```python
from build123d import *

# Parameters (mm, degrees)
F0_R     = 279.4
F1_DEPTH = 101.6
F2_R     = 12.7
F2_R_2   = 12.5
F3_DEPTH = 50.8


with BuildPart() as f1:
    # F0 (on Top) → F1 (new body)
    with BuildSketch(Plane.XY):
        with BuildLine():
            ThreePointArc((165.1, -285.961588), (285.961588, -165.1), (330.2, 0))
            ThreePointArc((330.2, 0), (316.035905, 95.673125), (274.758772, 183.138356))
            ThreePointArc((274.758772, 183.138356), (225.85856, 240.873309), (165.1, 285.961588))
            ThreePointArc((165.1, 285.961588), (-95.673125, 316.035905), (-295.981854, 146.378898))
            ThreePointArc((-295.981854, 146.378898), (-321.531685, 75.162596), (-330.2, 0))
            ThreePointArc((-330.2, 0), (-225.85856, -240.873309), (21.223083, -329.517254))
            ThreePointArc((21.223083, -329.517254), (95.673125, -316.035905), (165.1, -285.961588))
        make_face()
        Circle(F0_R, mode=Mode.SUBTRACT)
        with BuildLine():
            ThreePointArc((165.1, 285.961588), (225.85856, 240.873309), (274.758772, 183.138356))
            ThreePointArc((274.758772, 183.138356), (419.955029, 555.806639), (346.296428, 948.919871))
            ThreePointArc((346.296428, 948.919871), (343.096456, 900.151785), (327.593656, 853.80279))
            ThreePointArc((327.593656, 853.80279), (346.365994, 854.936106), (365.172292, 855.026849))
            Line((365.172292, 855.026849), (386.159106, 781.773906))
            ThreePointArc((386.159106, 781.773906), (330.519346, 792.374089), (274.106758, 787.298))
            ThreePointArc((274.106758, 787.298), (233.337853, 773.127606), (196.453349, 750.712498))
            ThreePointArc((196.453349, 750.712498), (183.140497, 739.629863), (170.813812, 727.459832))
            Line((170.813812, 727.459832), (159.193876, 746.42974))
            ThreePointArc((159.193876, 746.42974), (148.199724, 746.572871), (137.232142, 747.350049))
            ThreePointArc((137.232142, 747.350049), (210.182068, 520.220384), (165.1, 285.961588))
        make_face()
        with BuildLine():
            ThreePointArc((219.740654, 389.881855), (289.102738, 373.429577), (335.428058, 319.247098))
            Line((335.428058, 319.247098), (315.070275, 279.674231))
            ThreePointArc((315.070275, 279.674231), (278.207397, 339.338206), (208.315586, 345.151683))
            Line((208.315586, 345.151683), (219.740654, 389.881855))
        make_face(mode=Mode.SUBTRACT)
        with BuildLine():
            ThreePointArc((230.090316, 495.358171), (318.97663, 501.347432), (378.566059, 435.122451))
            Line((378.566059, 435.122451), (364.622182, 390.380044))
            ThreePointArc((364.622182, 390.380044), (308.575729, 448.660988), (227.861751, 443.851925))
            Line((227.861751, 443.851925), (230.090316, 495.358171))
        make_face(mode=Mode.SUBTRACT)
        with BuildLine():
            ThreePointArc((220.506904, 588.747772), (315.233937, 615.350933), (401.950913, 568.863247))
            Line((401.950913, 568.863247), (395.450001, 513.362684))
            ThreePointArc((395.450001, 513.362684), (315.191991, 550.934084), (228.323604, 533.417188))
            Line((228.323604, 533.417188), (220.506904, 588.747772))
        make_face(mode=Mode.SUBTRACT)
        with BuildLine():
            ThreePointArc((190.731506, 685.758289), (287.267753, 744.917108), (397.553807, 719.304627))
            Line((397.553807, 719.304627), (403.311044, 656.066156))
            ThreePointArc((403.311044, 656.066156), (302.181037, 674.537443), (211.661495, 625.806762))
            Line((211.661495, 625.806762), (190.731506, 685.758289))
        make_face(mode=Mode.SUBTRACT)
        with BuildLine():
            ThreePointArc((578.608057, -492.521545), (345.433034, -442.133203), (165.1, -285.961588))
            ThreePointArc((165.1, -285.961588), (95.673125, -316.035905), (21.223083, -329.517254))
            ThreePointArc((21.223083, -329.517254), (271.365154, -641.595043), (648.6405, -774.36144))
            ThreePointArc((648.6405, -774.36144), (608.006084, -747.206139), (575.618078, -710.605824))
            ThreePointArc((575.618078, -710.605824), (567.21339, -727.429803), (557.888826, -743.761906))
            Line((557.888826, -743.761906), (483.95651, -725.310549))
            ThreePointArc((483.95651, -725.310549), (520.956418, -682.425195), (544.76669, -631.032416))
            ThreePointArc((544.76669, -631.032416), (552.879221, -588.640311), (551.90942, -545.489839))
            ThreePointArc((551.90942, -545.489839), (548.968002, -528.419254), (544.591788, -511.659017))
            Line((544.591788, -511.659017), (566.830179, -511.080811))
            ThreePointArc((566.830179, -511.080811), (572.45121, -501.631161), (578.608057, -492.521545))
        make_face()
        with BuildLine():
            ThreePointArc((227.777264, -385.241916), (178.848131, -437.085104), (108.762068, -450.112768))
            Line((108.762068, -450.112768), (84.669851, -412.695977))
            ThreePointArc((84.669851, -412.695977), (154.771808, -410.603776), (194.752332, -352.982431))
            Line((194.752332, -352.982431), (227.777264, -385.241916))
        make_face(mode=Mode.SUBTRACT)
        with BuildLine():
            ThreePointArc((313.947602, -446.943144), (274.691297, -526.915581), (187.544067, -545.40905))
            Line((187.544067, -545.40905), (155.767944, -510.962094))
            ThreePointArc((155.767944, -510.962094), (234.263949, -491.564914), (270.456167, -419.260027))
            Line((270.456167, -419.260027), (313.947602, -446.943144))
        make_face(mode=Mode.SUBTRACT)
        with BuildLine():
            ThreePointArc((399.617075, -485.338467), (375.292572, -580.676064), (291.674567, -632.531325))
            Line((291.674567, -632.531325), (246.860125, -599.151088))
            ThreePointArc((246.860125, -599.151088), (319.526917, -548.431313), (347.791033, -464.442635))
            Line((347.791033, -464.442635), (399.617075, -485.338467))
        make_face(mode=Mode.SUBTRACT)
        with BuildLine():
            ThreePointArc((498.518346, -508.057474), (501.483263, -621.239726), (424.159177, -703.94401))
            Line((424.159177, -703.94401), (366.514436, -677.310688))
            ThreePointArc((366.514436, -677.310688), (433.076043, -598.965176), (436.133807, -496.207613))
            Line((436.133807, -496.207613), (498.518346, -508.057474))
        make_face(mode=Mode.SUBTRACT)
        with BuildLine():
            ThreePointArc((327.593656, 853.80279), (343.096456, 900.151785), (346.296428, 948.919871))
            ThreePointArc((346.296428, 948.919871), (23.952295, 1074.045306), (137.232142, 747.350049))
            ThreePointArc((137.232142, 747.350049), (148.199724, 746.572871), (159.193876, 746.42974))
            Line((159.193876, 746.42974), (140.616896, 776.757238))
            ThreePointArc((140.616896, 776.757238), (228.227479, 829.544451), (327.593656, 853.80279))
        make_face()
        Polygon((75.530644, 936.905829), (115.853144, 1006.746447), (196.498144, 1006.746447), (236.820644, 936.905829), (196.498144, 867.06521), (115.853144, 867.06521), align=None, mode=Mode.SUBTRACT)
        with BuildLine():
            ThreePointArc((648.6405, -774.36144), (918.174372, -557.765949), (578.608057, -492.521545))
            ThreePointArc((578.608057, -492.521545), (572.45121, -501.631161), (566.830179, -511.080811))
            Line((566.830179, -511.080811), (602.383053, -510.156423))
            ThreePointArc((602.383053, -510.156423), (604.292829, -612.42302), (575.618078, -710.605824))
            ThreePointArc((575.618078, -710.605824), (608.006084, -747.206139), (648.6405, -774.36144))
        make_face()
        Polygon((773.618927, -533.864371), (813.941427, -603.704989), (773.618927, -673.545608), (692.973927, -673.545608), (652.651427, -603.704989), (692.973927, -533.864371), align=None, mode=Mode.SUBTRACT)
        with BuildLine():
            ThreePointArc((-330.2, 0), (-321.531685, 75.162596), (-295.981854, 146.378898))
            ThreePointArc((-295.981854, 146.378898), (-691.320184, 85.788404), (-994.936929, -174.558431))
            ThreePointArc((-994.936929, -174.558431), (-951.102541, -152.945645), (-903.211734, -143.196967))
            ThreePointArc((-903.211734, -143.196967), (-913.579384, -127.506303), (-923.061118, -111.264943))
            Line((-923.061118, -111.264943), (-870.115616, -56.463358))
            ThreePointArc((-870.115616, -56.463358), (-851.475764, -109.948895), (-818.873448, -156.265585))
            ThreePointArc((-818.873448, -156.265585), (-786.217073, -184.487295), (-748.362768, -205.222658))
            ThreePointArc((-748.362768, -205.222658), (-732.108499, -211.210609), (-715.405601, -215.800815))
            Line((-715.405601, -215.800815), (-726.024055, -235.34893))
            ThreePointArc((-726.024055, -235.34893), (-720.650934, -244.94171), (-715.840199, -254.828503))
            ThreePointArc((-715.840199, -254.828503), (-555.615102, -78.087181), (-330.2, 0))
        make_face()
        with BuildLine():
            ThreePointArc((-689.249852, -177.700815), (-788.751016, -123.677382), (-821.712984, -15.360618))
            Line((-821.712984, -15.360618), (-769.82548, 21.244532))
            ThreePointArc((-769.82548, 21.244532), (-735.25708, -75.572267), (-647.795302, -129.59915))
            Line((-647.795302, -129.59915), (-689.249852, -177.700815))
        make_face(mode=Mode.SUBTRACT)
        with BuildLine():
            Line((-576.114637, -68.974553), (-620.12398, -103.409305))
            ThreePointArc((-620.12398, -103.409305), (-690.526509, -34.674869), (-693.62548, 63.668078))
            Line((-693.62548, 63.668078), (-642.310126, 85.788404))
            ThreePointArc((-642.310126, 85.788404), (-634.718908, -2.502771), (-576.114637, -68.974553))
        make_face(mode=Mode.SUBTRACT)
        with BuildLine():
            Line((-498.317918, -24.591898), (-544.037918, -48.415027))
            ThreePointArc((-544.037918, -48.415027), (-593.667927, 25.568149), (-566.110126, 110.286599))
            Line((-566.110126, 110.286599), (-520.390126, 120.582051))
            ThreePointArc((-520.390126, 120.582051), (-542.839678, 42.903926), (-498.317918, -24.591898))
        make_face(mode=Mode.SUBTRACT)
        with BuildLine():
            ThreePointArc((-447.517918, -4.639939), (-467.950869, 63.655527), (-444.190126, 130.86567))
            Line((-444.190126, 130.86567), (-399.740126, 133.021747))
            ThreePointArc((-399.740126, 133.021747), (-432.979205, 71.26557), (-403.067918, 7.830748))
            Line((-403.067918, 7.830748), (-447.517918, -4.639939))
        make_face(mode=Mode.SUBTRACT)
        with BuildLine():
            ThreePointArc((-903.211734, -143.196967), (-951.102541, -152.945645), (-994.936929, -174.558431))
            ThreePointArc((-994.936929, -174.558431), (-942.126667, -516.279357), (-715.840199, -254.828503))
            ThreePointArc((-715.840199, -254.828503), (-720.650934, -244.94171), (-726.024055, -235.34893))
            Line((-726.024055, -235.34893), (-742.999948, -266.600815))
            ThreePointArc((-742.999948, -266.600815), (-832.520308, -217.121431), (-903.211734, -143.196967))
        make_face()
        Polygon((-849.14957, -263.360221), (-808.82707, -333.200839), (-849.14957, -403.041458), (-929.79457, -403.041458), (-970.11707, -333.200839), (-929.79457, -263.360221), align=None, mode=Mode.SUBTRACT)
    extrude(amount=F1_DEPTH)

    # F2 (on face) → F3 (join)
    with BuildSketch(Plane(origin=(0, 0, 0), x_dir=(1, 0, 0), z_dir=(0, 0, -1))):
        with Locations((138.178983, 380.014748)):
            Circle(F2_R)
        with Locations((866.294952, 604.331288)):
            Circle(F2_R_2)
        with Locations((-956.513724, 448.067792)):
            Circle(F2_R_2)
        with Locations((90.218772, -1052.39908)):
            Circle(F2_R_2)
        with Locations((-398.191917, -70.340864)):
            Circle(F2_R)
        with Locations((260.012934, -309.673884)):
            Circle(F2_R)
    extrude(amount=F3_DEPTH)


solid = f1.part
```
Check sheet for the modelled part. Datum: model origin and axes. Units: mm. Give positions to 0.01 mm unless a question says otherwise; leave off trailing zeros. Order: outer loops, then holes, each group sorted by start corner. A loop starts at its lowest first (then second) coordinate and runs counter-clockwise, first axis right, second up. Notation, with made-up numbers: M 60,46 L 82,46 A21 cw 82,62 Z; hole C -25,-0.75 d11. An arc over 180 degrees is marked long. Answer in a Markdown table with one row per item.
1) Cross-section at B-B, the plane z = 28. Count the separate pieces of the cut face and the enclosed holes in it, plus the area to 3 significant figures.
Filled sheet:
| item | result |
|---|---|
| separate pieces | 1 |
| enclosed holes | 19 |
| area | 595,000 mm2 |
2) Cross-section at A-A, the plane x = -152. Enter the section's corners in (y, z), plus the area to 3 significant figures.
Filled sheet:
| item | result |
|---|---|
| outline | M -293.13,0 L -234.44,0 L -234.44,101.6 L -293.13,101.6 Z; M 234.44,0 L 293.13,0 L 293.13,101.6 L 234.44,101.6 Z |
| area | 11,900 mm2 |
3) Release check for a two-part mould opening along X. For faces 1 (the cylindrical face through (432.543, -600.332, 50.089)), 2 (the flat face through (216.94, 902.47, 50.09)) record: +X half, -X half, draft (parallel to the pull), parting line (faces both ways), or undercut.
Filled sheet:
| item | result |
|---|---|
| face 1 | undercut |
| face 2 | undercut |
4) Gauge pin test, flat ends, axial feed: P1, Ø2, axis at y = 265.5, z = 0, coming from the -X side; P2, Ø4, axis at y = -160, z = 57.5, coming from the +X side; P3, Ø2, axis at y = -447.5, z = 56, coming from the +X side. Record the tip position at first contact, or that the pin passes through.
Filled sheet:
| item | result |
|---|---|
| P1 | stops at x = -197.67 |
| P2 | stops at x = 289.94 |
| P3 | stops at x = 843.76 |
5) Thickness scan on L1, parallel to Y at x = 0, z = 47; L2, parallel to X at y = 298, z = 29; L3, parallel to Y at x = -881.5, z = 18. Record the ranges inside material, lowest first. Write a range as [from, to].
Filled sheet:
| item | result |
|---|---|
| L1 | y = [-330.2, -279.4], [279.4, 330.2], [827.82, 1045.99] |
| L2 | x = [-142.23, 142.23], [170.57, 311.23], [324.5, 346.26] |
| L3 | y = [-523.53, -403.04], [-263.36, -170.96], [-68.25, -41.04] |
